Design review of the part built by this model. Coordinates are the model's own, in mm. A direction names the side the tool comes from. Give positions to 0.01 mm unless a question says otherwise; leave off trailing zeros. Loops run counter-clockwise (first coordinate to the right, second up) from the corner with the lowest first, then second, coordinate; pieces in that order, holes last. Notation, with made-up numbers: M 61.5,-24 L 116.5,-24 A16 ccw 116.5,-12 Z; hole C 25.25,76 d1. An arc over 180 degrees is marked long. Use a Markdown table: item, result. Add a question column.
(1) For faces 5 (the face through (5.75, 5.79, 24.87)), 6 (the face through (-4.699, 0, 25)), list the 3-axis set-ups (+Z, -Z, +X, -X, +Y, -Y) from which the entire face can be reached by the end or side of a thin tool; tool diameter is ignored.
(2) Add section A-A, the plane z = 48. Give the boundary of the cut face in (x, y), then the cut area to 3 significant figures.
(3) Draft analysis for pull direction Y (two halves, no side actions). For faces 1 (the face through (-6.35, 0, 25)), 2 (the face through (4.699, 0, 25)), 3 (the face through (-5.75, -5.79, 24.87)), 4 (the face through (-5.79, 5.75, 24.87)), state which applies: pulls with the +Y half, pulls with the -Y half, needs draft (parallel to the pull), parting line crosses it, or undercut.
(4) Add section B-B, the plane x = 2. Give the boundary of the cut face in (y, z), then the cut area to 3 significant figures.
(5) For probe 1 along Y at (x, z) = (1, 49.5); probe 2 along X at (y, z) = (5, 37), list the stretches that pass through material, from the lowest coordinate up.
Autodesk Inventor part; units mm, degrees
ref_plane "Start plane" through (0, 0, -12.7) normal (0, 0, 1) x (1, 0, 0)
ref_plane "End plane" through (0, 0, 63.5) normal (0, 0, 1) x (1, 0, 0)
ref_plane "Work Plane4" through (6.35, -17.0688, -12.7) normal (0, 0, -1) x (-1, 0, 0)
ref_plane "Start plane" through (0, 0, -12.7) normal (0, 0, 1) x (1, 0, 0)
ref_plane "End plane" through (0, 0, 63.5) normal (0, 0, 1) x (1, 0, 0)
sketch "Sketch" plane through (0, 0, 0) normal (0, 0, 1) x (1, 0, 0)
  line L0 (-6.35, -4.3688) -> (-6.35, 4.3688)
  line L1 (-4.3688, 6.35) -> (4.3688, 6.35)
  line L2 (6.35, 4.3688) -> (6.35, -4.3688)
  line L3 (4.3688, -6.35) -> (-4.3688, -6.35)
  arc A0 (-6.35, -4.3688) -> (-4.3688, -6.35) centre (-4.3688, -4.3688) ccw
  arc A1 (-4.3688, 6.35) -> (-6.35, 4.3688) centre (-4.3688, 4.3688) ccw
  arc A2 (6.35, 4.3688) -> (4.3688, 6.35) centre (4.3688, 4.3688) ccw
  arc A3 (4.3688, -6.35) -> (6.35, -4.3688) centre (4.3688, -4.3688) ccw
  arc A4 (-4.3688, 4.699) -> (-4.699, 4.3688) centre (-4.3688, 4.3688) ccw
  line L4 (-4.3688, 4.699) -> (4.3688, 4.699)
  arc A5 (4.699, 4.3688) -> (4.3688, 4.699) centre (4.3688, 4.3688) ccw
  line L5 (4.699, 4.3688) -> (4.699, -4.3688)
  arc A6 (4.3688, -4.699) -> (4.699, -4.3688) centre (4.3688, -4.3688) ccw
  line L6 (4.3688, -4.699) -> (-4.3688, -4.699)
  arc A7 (-4.699, -4.3688) -> (-4.3688, -4.699) centre (-4.3688, -4.3688) ccw
  line L7 (-4.699, -4.3688) -> (-4.699, 4.3688)
  line L8 (0, 9.4644) -> (0, -9.4644) construction
  line L9 (-10.1124, 0) -> (13.3521, 0) construction
  dimension "d10" = 12.7
  dimension "d11" = 12.7
  dimension "d12" = 1.651
  dimension "d15" = 6.35
  dimension "d16" = 6.35
  dimension "d17" = 1.9812
extrude "Body" add sketch "Sketch" along normal up to surface (76.2 mm away) from surface at -12.7
sketch "Sketch3" plane through (0, 0, 0) normal (0, 0, 1) x (1, 0, 0)
  line L0 (0, 0) -> (10, 0)
ref_plane "Work Plane3" through (0, 0, 0) normal (0, -1, 0) x (1, 0, 0)
sketch "Sketch4" plane through (0, 0, 0) normal (0, -1, 0) x (1, 0, 0)
  line L0 (-2, -12.7) -> (12, -12.7)
  line L1 (-2, 63.5) -> (12, 63.5)
  dimension "d19" = 76.2
ref_plane "Work Plane4" through (6.35, -17.0688, -12.7) normal (0, 0, -1) x (-1, 0, 0)
split "Split1" plane through (6.35, -17.0688, -12.7) removes the side toward (0, 0, -1)
ref_plane "Work Plane5" through (6.35, -8.3312, 63.5) normal (0, 0, 1) x (1, 0, 0)
split "Split2" plane through (6.35, -8.3312, 63.5) removes the side toward (0, 0, 1)
equation "\"d10\" = G_H"
equation "\"d11\" = G_W"
equation "\"d12\" = G_T"
equation "\"d15\" = 0.5 * d10"
equation "\"d16\" = 0.5 * d11"
equation "\"d17\" = G_IR"
equation "\"d3\" = G_L"
equation "\"G_W\" = 12.7"
equation "\"G_H\" = 12.7"
equation "\"G_T\" = 1.651"
equation "\"G_IR\" = 1.2 * G_T"
equation "\"G_L\" = d19"
equation "\"G_OFFSET_START\" = 12.7"
equation "\"G_OFFSET_END\" = 12.7"
equation "\"d13\" = -G_OFFSET_START"
equation "\"d14\" = G_OFFSET_END + B_L"
equation "\"B_L\" = 50.8"
properties part number "ASTM A513 - 1/2 x 1/2 x 13/200 - 3" material "Steel, Mild"
Established:
| question | item | result |
|---|---|---|
| 1 | face 5 | +Z, -Z, +X, +Y |
| 1 | face 6 | +Z, -Z |
| 2 | outline | M -6.35,-4.37 A1.98 ccw -4.37,-6.35 L 4.37,-6.35 A1.98 ccw 6.35,-4.37 L 6.35,4.37 A1.98 ccw 4.37,6.35 L -4.37,6.35 A1.98 ccw -6.35,4.37 Z; hole M -4.7,-4.37 A0.33 ccw -4.37,-4.7 L 4.37,-4.7 A0.33 ccw 4.7,-4.37 L 4.7,4.37 A0.33 ccw 4.37,4.7 L -4.37,4.7 A0.33 ccw -4.7,4.37 Z |
| 2 | area | 69.7 mm^2 |
| 3 | face 1 | needs draft |
| 3 | face 2 | undercut |
| 3 | face 3 | pulls with the -Y half |
| 3 | face 4 | pulls with the +Y half |
| 4 | outline | M -6.35,-12.7 L -4.7,-12.7 L -4.7,63.5 L -6.35,63.5 Z; M 4.7,-12.7 L 6.35,-12.7 L 6.35,63.5 L 4.7,63.5 Z |
| 4 | area | 252 mm^2 |
| 5 | probe 1 | -6.35 to -4.7, 4.7 to 6.35 |
| 5 | probe 2 | -6.25 to 6.25 |
